Part print with two shaded views. Sizes in mm from the minimum x, y, z corner. A direction names the side the tool comes from. Round coordinates to 2 decimals unless told otherwise and drop trailing zeros. Write each loop counter-clockwise with the first axis right and the second up, starting at its lowest first coordinate (ties: lowest second). Pieces come first, ordered by that corner, then holes. Notation, with made-up numbers: (38, 82.5) -> (88, 82.5) arc R27 cw to (88, 101.5) -> close; hole circle Ø3 at (75, 81). An arc over 180 degrees is marked (long way). Answer in a Markdown table with one row per item.
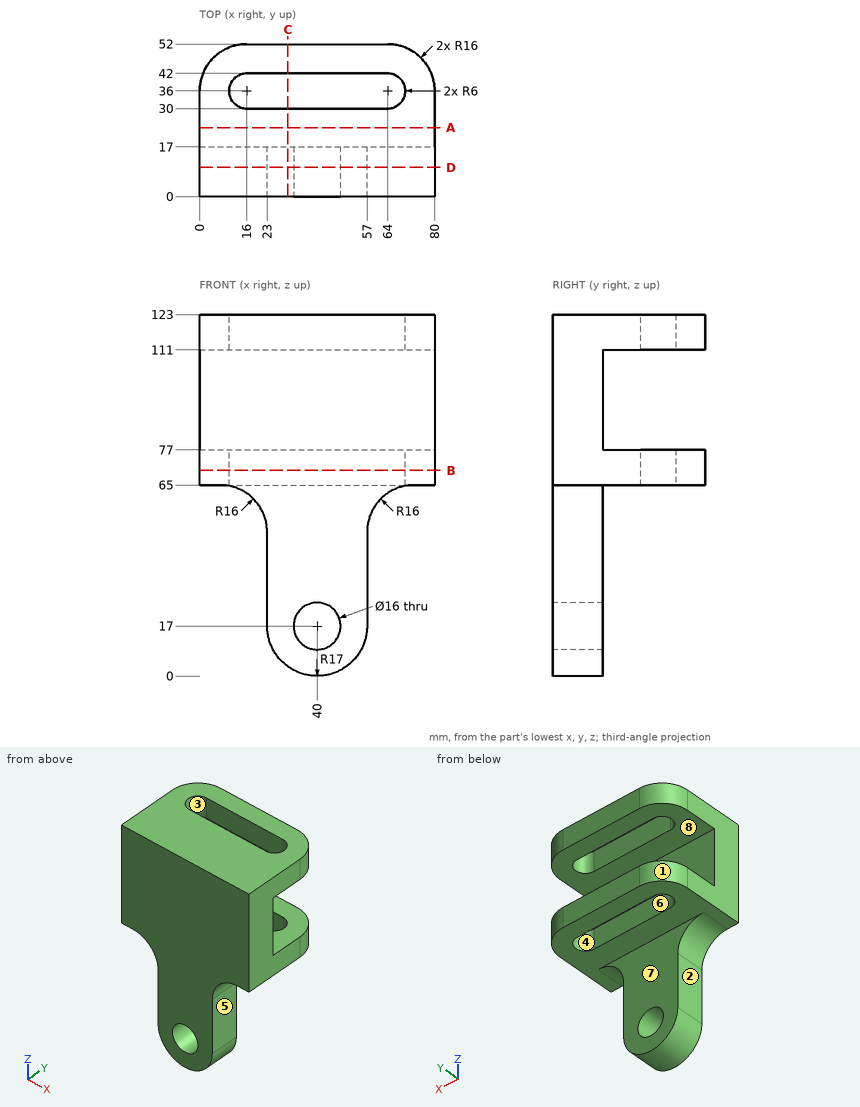
Q1. Saw through at B-B on z = 70. Write the cut outline in (x, y), plus the area to 3 significant figures.
A:
| item | result |
|---|---|
| outline | (0, 0) -> (80, 0) -> (80, 36) arc R16 ccw to (64, 52) -> (16, 52) arc R16 ccw to (0, 36) -> close; hole (16, 30) -> (64, 30) arc R6 ccw to (64, 42) -> (16, 42) arc R6 ccw to start |
| area | 3,360 mm² |
Q2. Which spindle directions (+Z, -Z, +X, -X, +Y, -Y) get a long thin tool onto all of the face, cutting with end or side? Do the marked faces 5, 6, 7 and 8. Say none if no direction does.
A:
| item | result |
|---|---|
| face 5 | -Z, +X, +Y, -Y |
| face 6 | +Z, -Z |
| face 7 | -Z, +X, -X, +Y |
| face 8 | +X, -X, +Y |
Q3. Saw through at C-C on x = 30. Write the cut outline in (y, z), plus the area to 3 significant figures.
A:
| item | result |
|---|---|
| outline | (0, 3.25) -> (17, 3.25) -> (17, 65) -> (30, 65) -> (30, 77) -> (17, 77) -> (17, 111) -> (30, 111) -> (30, 123) -> (0, 123) -> close; (42, 65) -> (52, 65) -> (52, 77) -> (42, 77) -> close; (42, 111) -> (52, 111) -> (52, 123) -> (42, 123) -> close |
| area | 2,590 mm² |
Q4. Two-plate mould, pull along Y, no slides. Class the marked faces 1, 2, 3 and 4: released by +Y, released by -Y, zero draft, split by the parting line, or undercut.
A:
| item | result |
|---|---|
| face 1 | released by +Y |
| face 2 | zero draft |
| face 3 | undercut |
| face 4 | undercut |
Q5. Wall check: line 1 (Z direction, x = 40, y = 9.5); line 2 (Y direction, x = 20, z = 71); line 3 (Z direction, x = 62, y = 47.5). Give the ranges that are in metal, low to high. Write a range as [from, to].
A:
| item | result |
|---|---|
| line 1 | [0, 9], [25, 123] |
| line 2 | [0, 30], [42, 52] |
| line 3 | [65, 77], [111, 123] |
Q6. Drop flat-ended pins along their axis: P1, Ø10, axis at x = 35.5, z = 89.5, coming from the +Y side; P2, Ø8.5, axis at y = 12.5, z = 36.5, coming from the +X side; P3, Ø1.5, axis at x = 22.5, y = 25, coming from the -Z side. Give the stop position or say it passes through.
A:
| item | result |
|---|---|
| P1 | y = 17 |
| P2 | x = 57 |
| P3 | z = 65 |
Q7. Saw through at A-A on y = 23.5. Write the cut outline in (x, z), plus the area to 3 significant figures.
A:
| item | result |
|---|---|
| outline | (0, 65) -> (80, 65) -> (80, 77) -> (0, 77) -> close; (0, 111) -> (80, 111) -> (80, 123) -> (0, 123) -> close |
| area | 1,920 mm² |
Q8. Saw through at D-D on y = 10. Write the cut outline in (x, z).
A:
| item | result |
|---|---|
| outline | (0, 65) -> (7, 65) arc R16 cw to (23, 49) -> (23, 17) arc R17 ccw to (57, 17) -> (57, 49) arc R16 cw to (73, 65) -> (80, 65) -> (80, 123) -> (0, 123) -> close; hole circle Ø16 at (40, 17) |
